```python
from build123d import *

# Parameters (mm, degrees)
FILLET_1_R          = 0.25
SKETCH_2_R          = 1.5
SKETCH_2_R_2        = 0.75
CUT_EXTRUDE_1_DEPTH = 0.5
CUT_EXTRUDE_2_REACH = 13.036
CUT_EXTRUDE_3_DEPTH = 0.5
CUT_EXTRUDE_4_DEPTH = 0.8
EXTRUDE_1_DEPTH     = 0.2


with BuildPart() as part:
    # Эскиз1 → Повернуть1 (revolve)
    with BuildSketch(Plane(origin=(0, 0, 0), x_dir=(1, 0, 0), z_dir=(0, 1, 0)), mode=Mode.PRIVATE) as revolve_1_sk:
        Polygon((0, 0), (0, -3.75), (-7, -3.75), (-7, -3.05), (-7.5, -3.05), (-7.5, -0.8), (-5.55, -0.8), (-5.55, 0), align=None)
    revolve(revolve_1_sk.sketch.rotate(Axis((0, 0, 0), (0, 0, -1)), 180), axis=Axis((0, 0, 0), (0, 0, -1)))

    # Скругление1
    fillet_1_edges = [part.edges().sort_by_distance(p)[0] for p in [
        (-5.55, 0, 0),
        (-7, 0, 3.75),
    ]]
    fillet(fillet_1_edges, radius=FILLET_1_R)

    # Эскиз2 → Вырез-Вытянуть1 (cut)
    with BuildSketch(Plane.XY.offset(3.75)):
        Circle(SKETCH_2_R)
        with Locations((0, -4)):
            Circle(SKETCH_2_R_2)
        with Locations((-3.464101615, -2)):
            Circle(SKETCH_2_R_2)
        with Locations((-3.464101615, 2)):
            Circle(SKETCH_2_R_2)
        with Locations((0, 4)):
            Circle(SKETCH_2_R_2)
        with Locations((3.464101615, 2)):
            Circle(SKETCH_2_R_2)
        with Locations((3.464101615, -2)):
            Circle(SKETCH_2_R_2)
    extrude(amount=-CUT_EXTRUDE_1_DEPTH, mode=Mode.SUBTRACT)

    # Эскиз3 → Вырез-Вытянуть2 (cut, up to next)
    with BuildSketch(Plane.XY.offset(3.05), mode=Mode.PRIVATE) as cut_extrude_2_sk1:
        with BuildLine():
            Line((0.5, -6.982120022), (0.5, -7.483314774))
            ThreePointArc((0.5, -7.483314774), (0, -7.5), (-0.5, -7.483314774))
            Line((-0.5, -7.483314774), (-0.5, -6.982120022))
            ThreePointArc((-0.5, -6.982120022), (0, -7), (0.5, -6.982120022))
        make_face()
    cut_extrude_2_tool1 = extrude(cut_extrude_2_sk1.sketch, amount=-CUT_EXTRUDE_2_REACH, mode=Mode.PRIVATE) & part.part
    add(cut_extrude_2_tool1.solids().sort_by_distance((0, -7.244238, 3.05))[0], mode=Mode.SUBTRACT)

    # Эскиз4 → Вырез-Вытянуть3 (cut)
    with BuildSketch(Plane(origin=(0, 0, 0.8), x_dir=(-1, 0, 0), z_dir=(0, 0, -1))):
        with BuildLine():
            Line((-4.751554754, -4.435394844), (-4.166748015, -3.889500094))
            ThreePointArc((-4.166748015, -3.889500094), (-5.421022143, -1.761396868), (-5.657160749, 0.697518642))
            Line((-5.657160749, 0.697518642), (-6.451148223, 0.795415996))
            ThreePointArc((-6.451148223, 0.795415996), (-6.181867356, -2.008610463), (-4.751554754, -4.435394844))
        make_face()
        with BuildLine():
            Line((-5.686622337, 3.148384728), (-4.986730357, 2.760891223))
            ThreePointArc((-4.986730357, 2.760891223), (-3.350375938, 4.611396868), (-1.084779161, 5.595824709))
            Line((-1.084779161, 5.595824709), (-1.237028868, 6.381203615))
            ThreePointArc((-1.237028868, 6.381203615), (-3.82060414, 5.258610463), (-5.686622337, 3.148384728))
        make_face()
        with BuildLine():
            Line((1.237028868, 6.381203615), (1.084779161, 5.595824709))
            ThreePointArc((1.084779161, 5.595824709), (3.350375938, 4.611396868), (4.986730357, 2.760891223))
            Line((4.986730357, 2.760891223), (5.686622337, 3.148384728))
            ThreePointArc((5.686622337, 3.148384728), (3.82060414, 5.258610463), (1.237028868, 6.381203615))
        make_face()
        with BuildLine():
            Line((6.451148223, 0.795415996), (5.657160749, 0.697518642))
            ThreePointArc((5.657160749, 0.697518642), (5.421022143, -1.761396868), (4.166748015, -3.889500094))
            Line((4.166748015, -3.889500094), (4.751554754, -4.435394844))
            ThreePointArc((4.751554754, -4.435394844), (6.181867356, -2.008610463), (6.451148223, 0.795415996))
        make_face()
    extrude(amount=-CUT_EXTRUDE_3_DEPTH, mode=Mode.SUBTRACT)

    # Эскиз5 → Вырез-Вытянуть4 (cut)
    with BuildSketch(Plane(origin=(0, 0, 0.8), x_dir=(-1, 0, 0), z_dir=(0, 0, -1))):
        with BuildLine():
            Line((-5, -5.590169944), (-3.7, -4.136725758))
            ThreePointArc((-3.7, -4.136725758), (0, -5.55), (3.7, -4.136725758))
            Line((3.7, -4.136725758), (5, -5.590169944))
            ThreePointArc((5, -5.590169944), (0, -7.5), (-5, -5.590169944))
        make_face()
    extrude(amount=-CUT_EXTRUDE_4_DEPTH, mode=Mode.SUBTRACT)

    # Эскиз6 → Бобышка-Вытянуть1 (add)
    with BuildSketch(Plane(origin=(0, 0, 1.6), x_dir=(-1, 0, 0), z_dir=(0, 0, -1))):
        with BuildLine():
            Line((-1.294304744, -6.904737521), (-1.110062076, -5.921856735))
            ThreePointArc((-1.110062076, -5.921856735), (-2.348915229, -5.548262994), (-3.479427056, -4.918761263))
            Line((-3.479427056, -4.918761263), (-4.056925322, -5.735153174))
            ThreePointArc((-4.056925322, -5.735153174), (-2.738776678, -6.46913652), (-1.294304744, -6.904737521))
        make_face()
        with BuildLine():
            Line((3.479427056, -4.918761263), (4.056925322, -5.735153174))
            ThreePointArc((4.056925322, -5.735153174), (2.738776678, -6.46913652), (1.294304744, -6.904737521))
            Line((1.294304744, -6.904737521), (1.110062076, -5.921856735))
            ThreePointArc((1.110062076, -5.921856735), (2.348915229, -5.548262994), (3.479427056, -4.918761263))
        make_face()
    extrude(amount=EXTRUDE_1_DEPTH)


solid = part.part
```
Input: part model. Units: mm. Frame: model coordinates. A direction names the side the tool comes from. Coordinates: 2 decimals unless noted, no trailing zeros. Write each loop counter-clockwise with the first axis right and the second up, starting at its lowest first coordinate (ties: lowest second). Pieces come first, ordered by that corner, then holes. Notation, with made-up numbers: (11, 27.25) - (47, 27.25) arc R10 cw to (47, 41.25) - close; hole circle Ø10 at (-15.5, -36). An arc over 180 degrees is marked (long way). Put each result on its own line as item: value. Start each with the question number.
1) Reachability of faces 1 (the face through (-1.5, 0.07, 3.5)), 2 (the face through (-5.43, -1.73, 1.05)) from +Z, -Z, +X, -X, +Y, -Y: full face, straight path, thin tool, end or side. Return the list, or none.
2) Cut plane A-A (y = 0). Return the cut outline in (x, z).
3) Mould query, pull axis X, two halves, no side actions, for faces 3 (the face through (-6, -2, 1.3)), 4 (the face through (-0.323, 7.493, 1.909)), 5 (the face through (0, 0, 0)). Classes: pulls with the +X half, pulls with the -X half, needs draft (parallel to the pull), parting line crosses it, or undercut.
4) Ray query, L1, parallel to Y at x = 0, z = 3.45; L2, parallel to Y at x = 0, z = 3.65; L3, parallel to Z at x = 0.5, y = 0.5. Return the intervals inside material, ascending.
5) Contact query for flat-ended pins moving along their axis: pin 1 (1 mm diameter, centred on x = -3, y = -6.5, fed in from -Z); pin 2 (1.1 mm diameter, centred on x = 4, y = 4, fed in from -Z); pin 3 (0.6 mm diameter, centred on y = -7, z = 2, fed in from +X); pin 4 (1.2 mm diameter, centred on x = 0, y = -4, fed in from +Z). Output: stop coordinate, or through.
6) Cut plane B-B (z = 2.5). Return the cut outline in (x, y).
Resolved:
1. face 1: +Z
1. face 2: -Z
2. outline: (-7.5, 0.8) - (-6.5, 0.8) - (-6.5, 1.3) - (-5.7, 1.3) - (-5.7, 0.8) - (-5.55, 0.8) - (-5.55, 0.25) arc R0.25 ccw to (-5.3, 0) - (5.3, 0) arc R0.25 ccw to (5.55, 0.25) - (5.55, 0.8) - (5.7, 0.8) - (5.7, 1.3) - (6.5, 1.3) - (6.5, 0.8) - (7.5, 0.8) - (7.5, 3.05) - (7, 3.05) - (7, 3.5) arc R0.25 ccw to (6.75, 3.75) - (1.5, 3.75) - (1.5, 3.25) - (-1.5, 3.25) - (-1.5, 3.75) - (-6.75, 3.75) arc R0.25 ccw to (-7, 3.5) - (-7, 3.05) - (-7.5, 3.05) - close
3. face 3: undercut
3. face 4: parting line crosses it
3. face 5: needs draft
4. L1: y = -7 to -4.75, -3.25 to -1.5, 1.5 to 3.25, 4.75 to 7
4. L2: y = -6.95 to -4.75, -3.25 to -1.5, 1.5 to 3.25, 4.75 to 6.95
4. L3: z = 0 to 3.25
5. pin 1: stops at z = 1.4
5. pin 2: stops at z = 0
5. pin 3: stops at x = 3.37
5. pin 4: stops at z = 3.25
6. outline: (-0.5, -7.48) - (-0.5, -6.98) arc R7 ccw to (0.5, -6.98) - (0.5, -7.48) arc R7.5 ccw (long way) to start
